Geometry check sheet. Reference: the model listing, model coordinates, mm. A direction names the side the tool comes from. Round coordinates to 2 decimals unless told otherwise and drop trailing zeros. Write each loop counter-clockwise with the first axis right and the second up, starting at its lowest first coordinate (ties: lowest second). Pieces come first, ordered by that corner, then holes. Notation, with made-up numbers: M 78.25,73.5 L 82.25,73.5 A11 cw 82.25,87.5 Z; hole C 47.25,18 d1. An arc over 180 degrees is marked long. One line per item, written item: value. Start each with the question number.
1. Depth check by flat-ended pin: P1, Ø6, axis at y = -22.5, z = 34.5, coming from the -X side; P2, Ø5.5, axis at x = 12.5, y = -16, coming from the +Z side; P3, Ø4, axis at x = 9.5, y = -10, coming from the +Z side. Enter the tip coordinate at first touch or a pass-through.
2. Section check A-A (x = 10). Record the boundary of the cut face in (y, z), and give its area (3 significant figures).
3. Access from +Z, -Z, +X, -X, +Y, -Y to the whole of each face (thin tool, end or side, straight path). Record for faces 4 (the flat face through (0, -19.05, 27)), 5 (the flat face through (0, 31.75, 19)).
4. Scan lines: probe 1 along Y at (x, z) = (20, 27); probe 2 along Y at (x, z) = (-27.5, 16.5); probe 3 along Y at (x, z) = (-11, 16). Record each from-to range of solid material in increasing order. Write a range as [from, to].
5. Release check for a two-part mould opening along Y. For faces 1 (the flat face through (-31.75, 0, 6)), 2 (the flat face through (0, -31.75, 19)), 3 (the flat face through (0, 19.05, 27)) record: pulls with the +Y half, pulls with the -Y half, needs draft (parallel to the pull), parting line crosses it, or undercut.
6. Section check D-D (z = 39). Record the boundary of the cut face in (x, y).
7. Section check C-C (y = -14). Record the boundary of the cut face in (x, z).
8. Section check B-B (z = 19). Record the boundary of the cut face in (x, y), and give its area (3 significant figures).
from build123d import *

# Parameters (mm, degrees)
F0_W     = 63.5
F0_H     = 63.5
F1_DEPTH = 12.7
F2_W     = 12.7
F2_H     = 38.1
F3_DEPTH = 63.5
F4_R     = 12.460297
F5_DEPTH = 63.5
F7_DEPTH = 63.5


with BuildPart() as f1:
    # F0 (on Top) → F1 (new body)
    with BuildSketch(Plane.XY):
        Rectangle(F0_W, F0_H)
    extrude(amount=F1_DEPTH)

    # F2 (on face) → F3 (join)
    with BuildSketch(Plane(origin=(-31.75, 0, 0), x_dir=(0, -1, 0), z_dir=(-1, 0, 0))):
        with Locations((-25.4, 31.75)):
            Rectangle(F2_W, F2_H)
        with Locations((25.4, 31.75)):
            Rectangle(F2_W, F2_H)
    extrude(amount=-F3_DEPTH)

    # F4 (on face) → F5 (join)
    with BuildSketch(Plane.YZ.offset(31.75)):
        with Locations((0, 12.724482)):
            Circle(F4_R)
    extrude(amount=-F5_DEPTH)

    # F6 (on face) → F7 (cut)
    with BuildSketch(Plane(origin=(0, 31.75, 0), x_dir=(-1, 0, 0), z_dir=(0, 1, 0))):
        Polygon((-31.75, 50.8), (-31.75, 10.989325), (-15.038024, 50.8), align=None)
        Polygon((15.038024, 50.8), (31.75, 10.989325), (31.75, 50.8), align=None)
    extrude(amount=-F7_DEPTH, mode=Mode.SUBTRACT)


solid = f1.part
Result sheet:
1. P1: stops at x = -23.14
1. P2: stops at z = 12.7
1. P3: stops at z = 22.28
2. outline: M -31.75,0 L 31.75,0 L 31.75,50.8 L 19.05,50.8 L 19.05,12.7 L 12.46,12.7 A12.46 ccw -12.46,12.7 L -19.05,12.7 L -19.05,50.8 L -31.75,50.8 Z
2. area: 2,020 mm2
3. face 4: +Z, +X, -X
3. face 5: +Z, -Z, +X, -X, +Y
4. probe 1: y = [-31.75, -19.05], [19.05, 31.75]
4. probe 2: y = [-31.75, -19.05], [-11.87, 11.87], [19.05, 31.75]
4. probe 3: y = [-31.75, -19.05], [-12.02, 12.02], [19.05, 31.75]
5. face 1: needs draft
5. face 2: pulls with the -Y half
5. face 3: undercut
6. outline: M -19.99,-31.75 L 19.99,-31.75 L 19.99,-19.05 L -19.99,-19.05 Z; M -19.99,19.05 L 19.99,19.05 L 19.99,31.75 L -19.99,31.75 Z
7. outline: M -31.75,0 L 31.75,0 L 31.75,10.99 L 31.03,12.7 L -31.03,12.7 L -31.75,10.99 Z
8. outline: M -28.39,-31.75 L 28.39,-31.75 L 28.39,-19.05 L -28.39,-19.05 Z; M -28.39,-10.76 L 28.39,-10.76 L 28.39,10.76 L -28.39,10.76 Z; M -28.39,19.05 L 28.39,19.05 L 28.39,31.75 L -28.39,31.75 Z
8. area: 2,660 mm2
